CAD build for the part. Positions are in the model's coordinates, mm. Face numbers are marked on the shaded views. A direction names the side the tool comes from. Give positions to 0.01 mm unless a question says otherwise; leave off trailing zeros. Write each loop counter-clockwise with the first axis right and the second up, starting at its lowest first coordinate (ties: lowest second). Pieces come first, ordered by that corner, then holes. Notation, with made-up numbers: (83, 42.5) -> (92, 42.5) arc R11 ccw to (92, 50.5) -> close; hole circle Ø6 at (33.5, -25). An arc over 180 degrees is marked (long way). Answer as a JSON object with one key per item and string values.
```python
from build123d import *

# Parameters (mm, degrees)
F0_R     = 22.5
F1_DEPTH = 25
F0_R_2   = 2.5
F2_DEPTH = 5
F3_R     = 30
F3_R_2   = 22.5
F4_DEPTH = 15
F5_SIZE  = 1
F6_SIZE  = 2


with BuildPart() as f1:
    # F0 (on Top) → F1 (new body)
    with BuildSketch(Plane.XY):
        with BuildLine():
            ThreePointArc((34.878679998, -2.9116458574), (34.9696568465, -1.4570861455), (35, 0))
            ThreePointArc((35, 0), (29.556068118, 18.7467020408), (14.9177807196, 31.6616458574))
            ThreePointArc((14.9177807196, 31.6616458574), (0, 35), (-14.9177807196, 31.6616458574))
            ThreePointArc((-14.9177807196, 31.6616458574), (-30.3108891325, 17.5), (-34.878679998, -2.9116458574))
            ThreePointArc((-34.878679998, -2.9116458574), (-30.3108891325, -17.5), (-19.9608992783, -28.75))
            ThreePointArc((-19.9608992783, -28.75), (0, -35), (19.9608992783, -28.75))
            ThreePointArc((19.9608992783, -28.75), (30.3108891325, -17.5), (34.878679998, -2.9116458574))
        make_face()
        Circle(F0_R, mode=Mode.SUBTRACT)
    extrude(amount=F1_DEPTH)

    # F0 (on Top) → F2 (join)
    with BuildSketch(Plane.XY):
        with BuildLine():
            ThreePointArc((-19.9608992783, -28.75), (-30.3108891325, -17.5), (-34.878679998, -2.9116458574))
            Line((-34.878679998, -2.9116458574), (-43.3012701892, -17.5))
            ThreePointArc((-43.3012701892, -17.5), (-43.3012701892, -25), (-36.8060796608, -28.75))
            Line((-36.8060796608, -28.75), (-19.9608992783, -28.75))
        make_face()
        with Locations((-36.8060796608, -21.25)):
            Circle(F0_R_2, mode=Mode.SUBTRACT)
        with BuildLine():
            Line((43.3012701892, -17.5), (34.878679998, -2.9116458574))
            ThreePointArc((34.878679998, -2.9116458574), (30.3108891325, -17.5), (19.9608992783, -28.75))
            Line((19.9608992783, -28.75), (36.8060796608, -28.75))
            ThreePointArc((36.8060796608, -28.75), (43.3012701892, -25), (43.3012701892, -17.5))
        make_face()
        with Locations((36.8060796608, -21.25)):
            Circle(F0_R_2, mode=Mode.SUBTRACT)
        with BuildLine():
            ThreePointArc((-14.9177807196, 31.6616458574), (0, 35), (14.9177807196, 31.6616458574))
            Line((14.9177807196, 31.6616458574), (6.4951905284, 46.25))
            ThreePointArc((6.4951905284, 46.25), (0, 50), (-6.4951905284, 46.25))
            Line((-6.4951905284, 46.25), (-14.9177807196, 31.6616458574))
        make_face()
        with Locations((0, 42.5)):
            Circle(F0_R_2, mode=Mode.SUBTRACT)
        with BuildLine():
            ThreePointArc((34.878679998, -2.9116458574), (34.9696568465, -1.4570861455), (35, 0))
            ThreePointArc((35, 0), (29.556068118, 18.7467020408), (14.9177807196, 31.6616458574))
            ThreePointArc((14.9177807196, 31.6616458574), (0, 35), (-14.9177807196, 31.6616458574))
            ThreePointArc((-14.9177807196, 31.6616458574), (-30.3108891325, 17.5), (-34.878679998, -2.9116458574))
            ThreePointArc((-34.878679998, -2.9116458574), (-30.3108891325, -17.5), (-19.9608992783, -28.75))
            ThreePointArc((-19.9608992783, -28.75), (0, -35), (19.9608992783, -28.75))
            ThreePointArc((19.9608992783, -28.75), (30.3108891325, -17.5), (34.878679998, -2.9116458574))
        make_face()
        Circle(F0_R, mode=Mode.SUBTRACT)
    extrude(amount=-F2_DEPTH)

    # F3 (on face) → F4 (join)
    with BuildSketch(Plane.XY.offset(25)):
        Circle(F3_R)
        Circle(F3_R_2, mode=Mode.SUBTRACT)
    extrude(amount=F4_DEPTH)

    # F5
    f5_edges = [f1.edges().sort_by_distance(p)[0] for p in [
        (-22.5, 0, 40),
        (-30, 0, 40),
        (34.87868, 2.911646, 25),
    ]]
    chamfer(f5_edges, length=F5_SIZE)

    # F6
    f6_edges = [f1.edges().sort_by_distance(p)[0] for p in [
        (-2.5, 42.5, 0),
        (34.30608, -21.25, 0),
        (-39.30608, -21.25, 0),
    ]]
    chamfer(f6_edges, length=F6_SIZE)


solid = f1.part
```
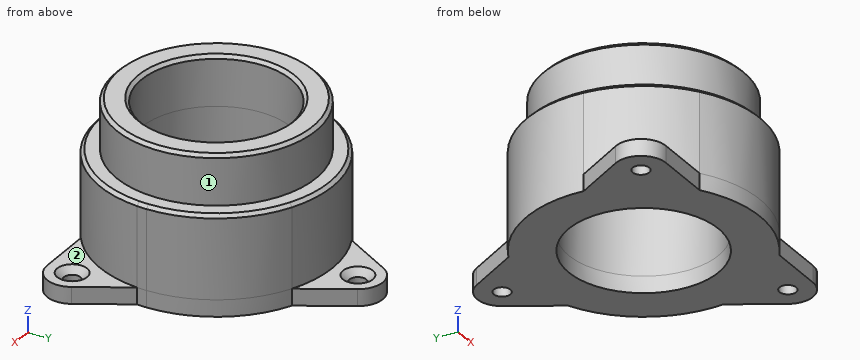
1) Slice it at A-A (x = 0). List the corners of the cut face in (y, z), then the cut area to 3 significant figures.
Model answer:
{"outline": "(-35, -5) -> (-22.5, -5) -> (-22.5, 39) -> (-23.5, 40) -> (-29, 40) -> (-30, 39) -> (-30, 25) -> (-34, 25) -> (-35, 24) -> close; (22.5, -5) -> (40, -5) -> (40, -2) -> (38, 0) -> (35, 0) -> (35, 24) -> (34, 25) -> (30, 25) -> (30, 39) -> (29, 40) -> (23.5, 40) -> (22.5, 39) -> close; (45, -5) -> (50, -5) -> (50, 0) -> (47, 0) -> (45, -2) -> close", "area": "1,020 mm2"}
2) Slice it at B-B (z = 21.5). List the corners of the cut face in (x, y).
Model answer:
{"outline": "circle Ø70 at (0, 0); hole circle Ø45 at (0, 0)"}
3) Pin check, flat tips, straight feed: pin 1 (9 mm diameter, centred on x = 0, y = 43, fed in from +Z); pin 2 (4.5 mm diameter, centred on x = -36.81, y = -21.25, fed in from -Z); pin 3 (10 mm diameter, centred on y = 3, z = 5.5, fed in from +X); pin 4 (4 mm diameter, centred on y = 16, z = 10, fed in from -X). Stop position of each tip, or through.
Model answer:
{"pin 1": "stops at z = 0", "pin 2": "passes through", "pin 3": "stops at x = 35", "pin 4": "stops at x = -32.08"}
4) Slice it at C-C (y = 42.5). List the corners of the cut face in (x, z).
Model answer:
{"outline": "(-8.66, -5) -> (-2.5, -5) -> (-2.5, -2) -> (-4.5, 0) -> (-8.66, 0) -> close; (2.5, -5) -> (8.66, -5) -> (8.66, 0) -> (4.5, 0) -> (2.5, -2) -> close"}
5) Wall check: probe 1 along Y at (x, z) = (0, -3.5); probe 2 along Y at (x, z) = (0, 32); probe 3 along Y at (x, z) = (0, 9). Give the ranges that are in metal, low to high.
Model answer:
{"probe 1": "y = -35 to -22.5, 22.5 to 40, 45 to 50", "probe 2": "y = -30 to -22.5, 22.5 to 30", "probe 3": "y = -35 to -22.5, 22.5 to 35"}
6) Slice it at D-D (y = -21.25). State how many separate pieces and enclosed holes the cut face has, then the cut area to 3 significant figures.
Model answer:
{"separate pieces": "4", "enclosed holes": "0", "area": "1,740 mm2"}
7) 3-axis set-ups, long thin cutter, end or side, ignore diameter. For the marked faces 1 and 2: which of +Z, -Z, +X, -X, +Y, -Y reach the whole face in a straight line?
Model answer:
{"face 1": "+Z", "face 2": "+Z, +X, -Y"}
